Part model, mm, in its own coordinate system. A direction names the side the tool comes from. Give positions to 0.01 mm unless a question says otherwise; leave off trailing zeros. Order: outer loops, then holes, each group sorted by start corner. A loop starts at its lowest first (then second) coordinate and runs counter-clockwise, first axis right, second up.
Autodesk Inventor part; units mm, degrees
ref_plane "YZ Plane" through (0, 0, 0) normal (1, 0, 0) x (0, 1, 0)
ref_plane "XZ Plane" through (0, 0, 0) normal (0, 1, 0) x (-1, 0, 0)
ref_plane "XY Plane" through (0, 0, 0) normal (0, 0, 1) x (1, 0, 0)
sketch "Sketch1" plane through (0, 0, 0) normal (0, 0, 1) x (1, 0, 0)
  line L0 (-7.5, 5) -> (7.5, 5)
  line L1 (7.5, 5) -> (7.5, -5)
  line L2 (7.5, -5) -> (-7.5, -5)
  line L3 (-7.5, -5) -> (-7.5, 5)
  line L4 (-7.5, 5) -> (7.5, -5) construction
  line L5 (7.5, 5) -> (-7.5, -5) construction
  line L6 (-7.5, 3.0607) -> (-6.4393, 2)
  line L7 (-7.5, 3.0607) -> (-6, 3.0607) construction
  line L8 (-6.4393, 2) -> (-7.5, 0.9393)
  line L9 (0, 5) -> (0, -5) construction
  line L10 (7.5, 3.0607) -> (6.4393, 2)
  line L11 (6.4393, 2) -> (7.5, 0.9393)
  point P0 (0, 0)
  point P1 (7.5, 0.9393)
  point P2 (7.5, 3.0607)
  dimension "d0" = 15
  dimension "d1" = 10
  dimension "d2" = 45
  dimension "d3" = 3
  dimension "d4" = 1.5
extrude "Extrusion1" add sketch "Sketch1" along normal mid plane 260 contours L0 L1 L10 L11 L2 L3 L8 L6
sketch "Sketch2" plane through (-7.5, 5, 130) normal (0, 1, 0) x (1, 0, 0)
  point P0 (7.5, 130)
  point P1 (7.5, 130)
hole "Hole1" at (0, 5, 0) direction (0, -1, 0) diameter 3.5 end through all counterbore diameter 6 counterbore depth 4.5
pattern_linear "Rectangular Pattern1" count 7 spacing 40 along (0, 0, 1) of "Hole1" first direction both ways yes
sketch "Sketch4" plane through (-7.5, 5, 130) normal (0, 1, 0) x (1, 0, 0)
  circle A0 centre (7.5, 250) radius 3
  circle A1 centre (7.5, 10) radius 3
  point P0 (7.5, 130)
hole "Hole3" at (0, 5, 120) at (0, 5, -120) direction (0, -1, 0) diameter 6 end through all
properties part number "MGN15 Rail Middle" material "Stainless Steel, 440C"
Item 1: Drop a flat-ended pin along its axis: P1, Ø3, axis at x = -1, z = 40.5, coming from the +Y side. Give the stop position or say it passes through.
Item 2: Pull direction X, two halves, no side cores. Call faces 1 (the face through (0, 0, 130)), 2 (the face through (0, 3, -43)), 3 (the face through (7.5, -2, -2)): released by +X, released by -X, zero draft, split by the parting line, or undercut.
Item 3: Band-saw the part on B-B on y = -1. List the corners of the cut face in (x, z).
Item 4: Which spindle directions (+Z, -Z, +X, -X, +Y, -Y) get a long thin tool onto all of the face, cutting with end or side? Do faces 4 (the face through (0, 3, 37)), 5 (the face through (-0.9, -0.07, 122.86)). Say none if no direction does.
Item 5: Drill centre lines: probe 1 along X at (y, z) = (3.35, -80); probe 2 along Z at (x, y) = (2, -0.25); probe 3 along X at (y, z) = (-3.35, -80). Where is each one in solid material? Low to high.
Item 6: Band-saw the part on A-A on z = -120. List the corners of the cut face in (x, y).
Item 7: Band-saw the part on C-C on z = 55.5. List the corners of the cut face in (x, y).
Working result:
1. P1: stops at y = 0.5
2. face 1: zero draft
2. face 2: undercut
2. face 3: released by +X
3. outline: (-7.5, -130) - (7.5, -130) - (7.5, 130) - (-7.5, 130) - close; hole circle Ø6 at (0, -120); hole circle Ø6 at (0, 120); hole circle Ø3.5 at (0, -80); hole circle Ø3.5 at (0, -40); hole circle Ø3.5 at (0, 0); hole circle Ø3.5 at (0, 40); hole circle Ø3.5 at (0, 80)
4. face 4: +Y
4. face 5: +Y, -Y
5. probe 1: x = -7.5 to -3, 3 to 7.5
5. probe 2: z = -130 to -122.24, -117.76 to 117.76, 122.24 to 130
5. probe 3: x = -7.5 to -1.75, 1.75 to 7.5
6. outline: (-7.5, -5) - (-3, -5) - (-3, 5) - (-7.5, 5) - (-7.5, 3.06) - (-6.44, 2) - (-7.5, 0.94) - close; (3, -5) - (7.5, -5) - (7.5, 0.94) - (6.44, 2) - (7.5, 3.06) - (7.5, 5) - (3, 5) - close
7. outline: (-7.5, -5) - (7.5, -5) - (7.5, 0.94) - (6.44, 2) - (7.5, 3.06) - (7.5, 5) - (-7.5, 5) - (-7.5, 3.06) - (-6.44, 2) - (-7.5, 0.94) - close
